```python
from build123d import *

# Parameters (mm, degrees)
BASE_FLANGE1_DEPTH           = 0.8
EDGE_FLANGE1_STRIP_W         = 5.2
EDGE_FLANGE1_STRIP_H         = 0.8
EDGE_FLANGE1_STRIP_CUT_DEPTH = 53
EDGE_FLANGE1_DEPTH           = 53
EDGE_FLANGE4_STRIP_W         = 5.2
EDGE_FLANGE4_STRIP_H         = 0.8
EDGE_FLANGE4_STRIP_CUT_DEPTH = 78
EDGE_FLANGE4_DEPTH           = 78
EDGE_FLANGE4_START           = 0.8
EDGE_FLANGE4_FLAT_DEPTH      = 0.8
EDGE_FLANGE6_STRIP_W         = 5.2
EDGE_FLANGE6_STRIP_H         = 0.8
EDGE_FLANGE6_STRIP_CUT_DEPTH = 69
EDGE_FLANGE6_DEPTH           = 69
EDGE_FLANGE6_PROFILE_W       = 69
EDGE_FLANGE6_PROFILE_H       = 9
EDGE_FLANGE6_FLAT_DEPTH      = 0.8
EDGE_FLANGE7_STRIP_W         = 5.2
EDGE_FLANGE7_STRIP_H         = 0.8
EDGE_FLANGE7_STRIP_CUT_DEPTH = 45
EDGE_FLANGE7_DEPTH           = 45
EDGE_FLANGE8_STRIP_W         = 5.2
EDGE_FLANGE8_STRIP_H         = 0.8
EDGE_FLANGE8_STRIP_CUT_DEPTH = 66
EDGE_FLANGE8_DEPTH           = 66
EDGE_FLANGE8_START           = 0.8
EDGE_FLANGE8_FLAT_DEPTH      = 0.8


# Sheet-metal steps are written as plain solids
with BuildPart() as part:
    # Sketch1 → Base-Flange1 (new body)
    with BuildSketch(Plane.XY.offset(20.561355821)):
        Polygon((22.147479573, -45.981220417), (-23.852520427, -45.981220417), (-23.852520427, -20.981220417), (-45.852520427, -20.981220417), (-45.852520427, 32.018779583), (22.147479573, 32.018779583), align=None)
    extrude(amount=BASE_FLANGE1_DEPTH)

    # Edge-Flange1 strip (across the edge) → Edge-Flange1 strip cut (cut)
    with BuildSketch(Plane(origin=(-45.852520427, -20.981220417, 20.561355821), x_dir=(1, 0, 0), z_dir=(0, 1, 0))):
        with Locations((-1.6, -0.4)):
            Rectangle(EDGE_FLANGE1_STRIP_W, EDGE_FLANGE1_STRIP_H)
    extrude(amount=EDGE_FLANGE1_STRIP_CUT_DEPTH, mode=Mode.SUBTRACT)

    # Edge-Flange1 section (across the edge) → Edge-Flange1 (add)
    with BuildSketch(Plane(origin=(-45.852520427, -20.981220417, 20.561355821), x_dir=(1, 0, 0), z_dir=(0, 1, 0))):
        with BuildLine():
            Line((-0.8, 1), (-0.8, 18))
            Line((-0.8, 18), (0, 18))
            Line((0, 18), (0, 1))
            ThreePointArc((0, 1), (0.292893219, 0.292893219), (1, 0))
            Line((1, 0), (1, -0.8))
            ThreePointArc((1, -0.8), (-0.272792206, -0.272792206), (-0.8, 1))
        make_face()
    extrude(amount=EDGE_FLANGE1_DEPTH)

    # Edge-Flange4 strip (across the edge) → Edge-Flange4 strip cut (cut)
    with BuildSketch(Plane(origin=(22.147479573, 32.018779583, 20.561355821), x_dir=(-1, 0, 0), z_dir=(0, -1, 0))):
        with Locations((-1.6, -0.4)):
            Rectangle(EDGE_FLANGE4_STRIP_W, EDGE_FLANGE4_STRIP_H)
    extrude(amount=EDGE_FLANGE4_STRIP_CUT_DEPTH, mode=Mode.SUBTRACT)

    # Edge-Flange4 bend section (across the edge) → Edge-Flange4 (add)
    with BuildSketch(Plane(origin=(22.147479573, 32.018779583, 20.561355821), x_dir=(-1, 0, 0), z_dir=(0, -1, 0))):
        with BuildLine():
            Line((-0.8, 1), (0, 1))
            ThreePointArc((0, 1), (0.292893219, 0.292893219), (1, 0))
            Line((1, 0), (1, -0.8))
            ThreePointArc((1, -0.8), (-0.272792206, -0.272792206), (-0.8, 1))
        make_face()
    extrude(amount=EDGE_FLANGE4_DEPTH)

    # Edge-Flange4 profile (on flange) → Edge-Flange4 flat (add)
    with BuildSketch(Plane(origin=(22.147479573, 0, 20.561355821), x_dir=(0, -1, 0), z_dir=(1, 0, 0)).offset(EDGE_FLANGE4_START)):
        Polygon((45.981220417, 1), (45.981220417, 20), (43.981220417, 20), (43.981220417, 21), (-25.018779583, 21), (-25.018779583, 20), (-32.018779583, 20), (-32.018779583, 1), align=None)
    extrude(amount=-EDGE_FLANGE4_FLAT_DEPTH)

    # Edge-Flange6 strip (across the edge) → Edge-Flange6 strip cut (cut)
    with BuildSketch(Plane(origin=(22.947479573, -43.981220417, -0.438644179), x_dir=(0, 0, 1), z_dir=(0, 1, 0))):
        with Locations((-0.8, -0.4)):
            Rectangle(EDGE_FLANGE6_STRIP_W, EDGE_FLANGE6_STRIP_H)
    extrude(amount=EDGE_FLANGE6_STRIP_CUT_DEPTH, mode=Mode.SUBTRACT)

    # Edge-Flange6 bend section (across the edge) → Edge-Flange6 (add)
    with BuildSketch(Plane(origin=(22.947479573, -43.981220417, -0.438644179), x_dir=(0, 0, 1), z_dir=(0, 1, 0))):
        with BuildLine():
            Line((0, 1), (0.8, 1))
            ThreePointArc((0.8, 1), (1.092893219, 0.292893219), (1.8, 0))
            Line((1.8, 0), (1.8, -0.8))
            ThreePointArc((1.8, -0.8), (0.527207794, -0.272792206), (0, 1))
        make_face()
    extrude(amount=EDGE_FLANGE6_DEPTH)

    # Edge-Flange6 profile (on flange) → Edge-Flange6 flat (add)
    with BuildSketch(Plane(origin=(22.947479573, 0, -0.438644179), x_dir=(0, 1, 0), z_dir=(0, 0, -1))):
        with Locations((-9.481220417, 5.5)):
            Rectangle(EDGE_FLANGE6_PROFILE_W, EDGE_FLANGE6_PROFILE_H)
        with BuildLine():
            Line((-25.581220417, 3.3), (-25.581220417, 7.3))
            ThreePointArc((-25.581220417, 7.3), (-23.981220417, 8.9), (-22.381220417, 7.3))
            Line((-22.381220417, 7.3), (-22.381220417, 3.3))
            ThreePointArc((-22.381220417, 3.3), (-23.981220417, 1.7), (-25.581220417, 3.3))
        make_face(mode=Mode.SUBTRACT)
        with BuildLine():
            ThreePointArc((9.418779583, 7.3), (11.018779583, 8.9), (12.618779583, 7.3))
            Line((12.618779583, 7.3), (12.618779583, 3.3))
            ThreePointArc((12.618779583, 3.3), (11.018779583, 1.7), (9.418779583, 3.3))
            Line((9.418779583, 3.3), (9.418779583, 7.3))
        make_face(mode=Mode.SUBTRACT)
    extrude(amount=-EDGE_FLANGE6_FLAT_DEPTH)

    # Edge-Flange7 strip (across the edge) → Edge-Flange7 strip cut (cut)
    with BuildSketch(Plane(origin=(21.147479573, -45.981220417, 20.561355821), x_dir=(0, 1, 0), z_dir=(-1, 0, 0))):
        with Locations((-1.6, -0.4)):
            Rectangle(EDGE_FLANGE7_STRIP_W, EDGE_FLANGE7_STRIP_H)
    extrude(amount=EDGE_FLANGE7_STRIP_CUT_DEPTH, mode=Mode.SUBTRACT)

    # Edge-Flange7 section (across the edge) → Edge-Flange7 (add)
    with BuildSketch(Plane(origin=(21.147479573, -45.981220417, 20.561355821), x_dir=(0, 1, 0), z_dir=(-1, 0, 0))):
        with BuildLine():
            Line((-0.8, 1), (-0.8, 21))
            Line((-0.8, 21), (0, 21))
            Line((0, 21), (0, 1))
            ThreePointArc((0, 1), (0.292893219, 0.292893219), (1, 0))
            Line((1, 0), (1, -0.8))
            ThreePointArc((1, -0.8), (-0.272792206, -0.272792206), (-0.8, 1))
        make_face()
    extrude(amount=EDGE_FLANGE7_DEPTH)

    # Edge-Flange8 strip (across the edge) → Edge-Flange8 strip cut (cut)
    with BuildSketch(Plane(origin=(-44.852520427, 32.018779583, 20.561355821), x_dir=(0, -1, 0), z_dir=(1, 0, 0))):
        with Locations((-1.6, -0.4)):
            Rectangle(EDGE_FLANGE8_STRIP_W, EDGE_FLANGE8_STRIP_H)
    extrude(amount=EDGE_FLANGE8_STRIP_CUT_DEPTH, mode=Mode.SUBTRACT)

    # Edge-Flange8 bend section (across the edge) → Edge-Flange8 (add)
    with BuildSketch(Plane(origin=(-44.852520427, 32.018779583, 20.561355821), x_dir=(0, -1, 0), z_dir=(1, 0, 0))):
        with BuildLine():
            Line((-0.8, 1), (0, 1))
            ThreePointArc((0, 1), (0.292893219, 0.292893219), (1, 0))
            Line((1, 0), (1, -0.8))
            ThreePointArc((1, -0.8), (-0.272792206, -0.272792206), (-0.8, 1))
        make_face()
    extrude(amount=EDGE_FLANGE8_DEPTH)

    # Edge-Flange8 profile (on flange) → Edge-Flange8 flat (add)
    with BuildSketch(Plane(origin=(0, 32.018779583, 20.561355821), x_dir=(1, 0, 0), z_dir=(0, 1, 0)).offset(EDGE_FLANGE8_START)):
        Polygon((21.147479573, 1), (21.147479573, 21), (-6.852520427, 21), (-6.852520427, 5), (-28.852520427, 5), (-28.852520427, 21), (-44.852520427, 21), (-44.852520427, 1), align=None)
    extrude(amount=-EDGE_FLANGE8_FLAT_DEPTH)


solid = part.part
```
Geometry: final body of the model. Coordinates: model frame, mm. A direction names the side the tool comes from. Give positions to 0.01 mm unless a question says otherwise; leave off trailing zeros. Loops run counter-clockwise (first coordinate to the right, second up) from the corner with the lowest first, then second, coordinate; pieces in that order, holes last. Notation, with made-up numbers: (54.25, -34.5) -> (72.25, -34.5) arc R12 cw to (72.25, -28.5) -> close; hole circle Ø4 at (21.5, -17). An arc over 180 degrees is marked (long way). Use CSV: the item, a comma, the result in double quotes.
(1) Cut plane D-D (x = -36). Output: boundary loops of the cut face in (y, z), plus the area to 3 significant figures.
From the geometry:
outline,"(-20.98, 20.56) -> (31.02, 20.56) arc R1 cw to (32.02, 19.56) -> (32.02, -0.44) -> (32.82, -0.44) -> (32.82, 19.56) arc R1.8 ccw to (31.02, 21.36) -> (-20.98, 21.36) -> close"
area,"59.4 mm^2"
(2) First-contact query: P1, Ø9.5, axis at x = -37.5, z = 12, coming from the -Y side; P2, Ø0.9, axis at x = 22, z = 12, coming from the +Y side; P3, Ø5, axis at y = 4, z = 14.5, coming from the +X side. Flat tips, straight axial feed; report the tip coordinate or a pass-through.
From the geometry:
P1,"y = 32.02"
P2,"y = 32.02"
P3,"x = 22.95"
(3) Cut plane A-A (z = 5.25). Output: boundary loops of the cut face in (x, y), plus the area to 3 significant figures.
From the geometry:
outline,"(-46.65, -20.98) -> (-45.85, -20.98) -> (-45.85, 32.02) -> (-46.65, 32.02) -> close; (-44.85, 32.02) -> (-28.85, 32.02) -> (-28.85, 32.82) -> (-44.85, 32.82) -> close; (-23.85, -46.78) -> (21.15, -46.78) -> (21.15, -45.98) -> (-23.85, -45.98) -> close; (-6.85, 32.02) -> (21.15, 32.02) -> (21.15, 32.82) -> (-6.85, 32.82) -> close; (22.15, -45.98) -> (22.95, -45.98) -> (22.95, 32.02) -> (22.15, 32.02) -> close"
area,"176 mm^2"
(4) Cut plane B-B (y = -35.5). Output: boundary loops of the cut face in (x, z).
From the geometry:
outline,"(-23.85, 20.56) -> (21.15, 20.56) arc R1 cw to (22.15, 19.56) -> (22.15, 1.36) arc R1.8 ccw to (23.95, -0.44) -> (32.95, -0.44) -> (32.95, 0.36) -> (23.95, 0.36) arc R1 cw to (22.95, 1.36) -> (22.95, 19.56) arc R1.8 ccw to (21.15, 21.36) -> (-23.85, 21.36) -> close"
(5) Pull-direction query (X, two-part tool) for faces 4 (the face through (-1.04, -46.24, 20.85)), 5 (the face through (-46.653, 5, 11)), 6 (the face through (-45.853, 5, 11)); classes: released by +X, released by -X, zero draft, split by the parting line, or undercut.
From the geometry:
face 4,"zero draft"
face 5,"released by -X"
face 6,"undercut"
(6) Access query for faces 1 (the face through (-12.315, 32.278, 20.848)), 2 (the face through (-1, -45.981, 9)), 3 (the face through (-5, 32.019, 9)). Directions: +Z, -Z, +X, -X, +Y, -Y. A direction counts if a zero-diameter tool reaches every point of the face in a straight line with its end or side. Return the directions, or none.
From the geometry:
face 1,"+Z, +Y"
face 2,"-Z, -X"
face 3,"-Z"
(7) Cut plane C-C (z = 16.5). Output: boundary loops of the cut face in (x, y).
From the geometry:
outline,"(-46.65, -20.98) -> (-45.85, -20.98) -> (-45.85, 32.02) -> (-46.65, 32.02) -> close; (-44.85, 32.02) -> (21.15, 32.02) -> (21.15, 32.82) -> (-44.85, 32.82) -> close; (-23.85, -46.78) -> (21.15, -46.78) -> (21.15, -45.98) -> (-23.85, -45.98) -> close; (22.15, -45.98) -> (22.95, -45.98) -> (22.95, 32.02) -> (22.15, 32.02) -> close"
(8) Ray query, line 1 along Y through (x, z) = (9.5, 7.5); line 2 along X through (y, z) = (3, 15.25); line 3 along Y through (x, z) = (-17, 8.5). Return the intervals inside material, ascending. Write a range as [from, to].
From the geometry:
line 1,"[-46.78, -45.98], [32.02, 32.82]"
line 2,"[-46.65, -45.85], [22.15, 22.95]"
line 3,"[-46.78, -45.98]"
